```python
from build123d import *

# Parameters (mm, degrees)
SKETCH_1_W          = 120
SKETCH_1_H          = 120
EXTRUDE_1_DEPTH     = 3
SKETCH_3_W          = 123
SKETCH_3_H          = 120
EXTRUDE_2_DEPTH     = 5
SKETCH_5_W          = 15.3
SKETCH_5_H          = 15
CUT_EXTRUDE_2_DEPTH = 3
SKETCH_6_R          = 2.6
CUT_EXTRUDE_3_DEPTH = 87.291656607
SKETCH_7_R          = 5.5
CUT_EXTRUDE_4_DEPTH = 1
SKETCH_8_W          = 92.4
SKETCH_8_H          = 3
CUT_EXTRUDE_5_DEPTH = 3
SKETCH_9_R          = 0.5
CUT_EXTRUDE_6_DEPTH = 3
FILLET_1_R          = 1
FILLET_2_R          = 0.5


with BuildPart() as part:
    # 草图1 → 凸台-拉伸1 (new body)
    with BuildSketch(Plane(origin=(0, 0, 0), x_dir=(1, 0, 0), z_dir=(0, 1, 0))):
        Rectangle(SKETCH_1_W, SKETCH_1_H)
    extrude(amount=EXTRUDE_1_DEPTH)

    # 草图3 → 凸台-拉伸2 (add)
    with BuildSketch(Plane.XZ):
        Rectangle(SKETCH_3_W, SKETCH_3_H)
    extrude(amount=EXTRUDE_2_DEPTH)

    # 草图5 → 切除-拉伸2 (cut)
    with BuildSketch(Plane(origin=(0, 3, 0), x_dir=(1, 0, 0), z_dir=(0, 1, 0))):
        with Locations((-53.85, 52.5)):
            Rectangle(SKETCH_5_W, SKETCH_5_H)
        with Locations((53.85, 52.5)):
            Rectangle(SKETCH_5_W, SKETCH_5_H)
        with Locations((-53.85, -52.5)):
            Rectangle(SKETCH_5_W, SKETCH_5_H)
        with Locations((53.85, -52.5)):
            Rectangle(SKETCH_5_W, SKETCH_5_H)
    extrude(amount=-CUT_EXTRUDE_2_DEPTH, mode=Mode.SUBTRACT)

    # 草图6 → 切除-拉伸3 (cut, through all)
    with BuildSketch(Plane(origin=(0, 3, 0), x_dir=(1, 0, 0), z_dir=(0, 1, 0))):
        with Locations(Location((-53.85, 52.5, 0), (0, 0, 270))):
            Circle(SKETCH_6_R)
        with Locations(Location((53.85, 52.5, 0), (0, 0, 270))):
            Circle(SKETCH_6_R)
        with Locations(Location((-53.85, -52.5, 0), (0, 0, 270))):
            Circle(SKETCH_6_R)
        with Locations(Location((53.85, -52.5, 0), (0, 0, 270))):
            Circle(SKETCH_6_R)
    extrude(amount=-CUT_EXTRUDE_3_DEPTH, mode=Mode.SUBTRACT)

    # 草图7 → 切除-拉伸4 (cut)
    with BuildSketch(Plane.XZ.offset(5)):
        with Locations(Location((-53.85, 52.5, 0), (0, 0, 270))):
            Circle(SKETCH_7_R)
        with Locations(Location((-53.85, -52.5, 0), (0, 0, 270))):
            Circle(SKETCH_7_R)
        with Locations(Location((53.85, 52.5, 0), (0, 0, 270))):
            Circle(SKETCH_7_R)
        with Locations(Location((53.85, -52.5, 0), (0, 0, 270))):
            Circle(SKETCH_7_R)
    extrude(amount=-CUT_EXTRUDE_4_DEPTH, mode=Mode.SUBTRACT)

    # 草图8 → 切除-拉伸5 (cut)
    with BuildSketch(Plane(origin=(0, 3, 0), x_dir=(1, 0, 0), z_dir=(0, 1, 0))):
        with Locations((0, 58.5)):
            Rectangle(SKETCH_8_W, SKETCH_8_H)
        with Locations((0, -58.5)):
            Rectangle(SKETCH_8_W, SKETCH_8_H)
    extrude(amount=-CUT_EXTRUDE_5_DEPTH, mode=Mode.SUBTRACT)

    # 草图9 → 切除-拉伸6 (cut)
    with BuildSketch(Plane(origin=(0, 3, 0), x_dir=(1, 0, 0), z_dir=(0, 1, 0))):
        with Locations((-46.7, 45)):
            Circle(SKETCH_9_R)
        with Locations((46.7, 45)):
            Circle(SKETCH_9_R)
        with Locations((-46.7, -45)):
            Circle(SKETCH_9_R)
        with Locations((46.7, -45)):
            Circle(SKETCH_9_R)
    extrude(amount=-CUT_EXTRUDE_6_DEPTH, mode=Mode.SUBTRACT)

    # 圆角1
    fillet_1_edges = [part.edges().sort_by_distance(p)[0] for p in [
        (47.2, 1.5, -45),
        (-47.2, 1.5, 45),
        (47.2, 1.5, 45),
        (-47.2, 1.5, -45),
    ]]
    fillet(fillet_1_edges, radius=FILLET_1_R)

    # 圆角2
    fillet_2_edges = [part.edges().sort_by_distance(p)[0] for p in [
        (46.2, 1.5, -57),
        (-46.2, 1.5, -57),
        (-46.2, 1.5, 57),
        (46.2, 1.5, 57),
        (60, 1.5, -45),
        (-60, 1.5, 45),
        (60, 1.5, 45),
        (-60, 1.5, -45),
    ]]
    fillet(fillet_2_edges, radius=FILLET_2_R)


solid = part.part
```
For this review, take the finished solid that the model builds, in its own axes (mm). A direction names the side the tool comes from. Coordinates: 2 decimals unless noted, no trailing zeros. Loops run counter-clockwise (first coordinate to the right, second up) from the corner with the lowest first, then second, coordinate; pieces in that order, holes last. Notation, with made-up numbers: (54.25, 74.5) -> (104.25, 74.5) arc R8 ccw to (104.25, 85.5) -> close; hole circle Ø2 at (8, -37.75). An arc over 180 degrees is marked (long way). Return JSON: item names as keys, results as strings. Group by question number.
(1) Consider section C-C, the plane x = 13.5. Give the boundary of the cut face in (y, z), plus the area to 3 significant figures.
(2) Mouldability with a two-part tool opening along Z and no side actions: class faces 5 (the flat face through (-61.5, -2, -1)), 6 (the flat face through (-54, 2, 45)), 7 (the flat face through (51, -4, -54)) as pulls with the +Z half, pulls with the -Z half, needs draft (parallel to the pull), parting line crosses it, or undercut.
(3) Tool access review of faces 1 (the flat face through (51, -4, 51)), 2 (the flat face through (46.2, 2, 51)), 3 (the flat face through (-1, 2, 57)), 4 (the flat face through (-60, 1, 1)): name each direction out of +Z, -Z, +X, -X, +Y, -Y from which nothing blocks a thin tool from reaching the whole face with its end or side.
(4) Consider section B-B, the plane z = -52. Give the boundary of the cut face in (x, y), plus the area to 3 significant figures.
(5) Consider section A-A, the plane x = 53.85. Give the boundary of the cut face in (y, z).
(6) To check wall thickness, follow L1, parallel to X at y = -2, z = -52.5; L2, parallel to X at y = -4.65, z = 52.5; L3, parallel to Z at x = -54.5, y = -3.25. State the ranges of each line that lie inside material, in increasing order.
(7) For pin 1 Ø0.9 at (y, z) = (2, -16) entering from +X; pin 2 Ø9 at (x, z) = (53.85, -52.5) entering from -Y; pin 3 Ø2.5 at (y, z) = (2, -51.5) entering from -X, all flat-tipped, find the tip position at first contact; note any pin that passes through.
Results below:
{
 "1": {"outline": "(-5, -60) -> (0, -60) -> (0, -57) -> (3, -57) -> (3, 57) -> (0, 57) -> (0, 60) -> (-5, 60) -> close", "area": "942 mm2"},
 "2": {"face 5": "needs draft", "face 6": "pulls with the +Z half", "face 7": "undercut"},
 "3": {"face 1": "-Y", "face 2": "+Z, +X, +Y", "face 3": "+Z, +X, -X, +Y", "face 4": "+Z, -Z, -X, +Y"},
 "4": {"outline": "(-61.5, -5) -> (-59.33, -5) -> (-59.33, -4) -> (-56.4, -4) -> (-56.4, 0) -> (-61.5, 0) -> close; (-51.3, -4) -> (-48.37, -4) -> (-48.37, -5) -> (48.37, -5) -> (48.37, -4) -> (51.3, -4) -> (51.3, 0) -> (46.2, 0) -> (46.2, 3) -> (-46.2, 3) -> (-46.2, 0) -> (-51.3, 0) -> close; (56.4, -4) -> (59.33, -4) -> (59.33, -5) -> (61.5, -5) -> (61.5, 0) -> (56.4, 0) -> close", "area": "829 mm2"},
 "5": {"outline": "(-5, -60) -> (0, -60) -> (0, -55.1) -> (-4, -55.1) -> (-4, -58) -> (-5, -58) -> close; (-5, -47) -> (-4, -47) -> (-4, -49.9) -> (0, -49.9) -> (0, -45) -> (3, -45) -> (3, 45) -> (0, 45) -> (0, 49.9) -> (-4, 49.9) -> (-4, 47) -> (-5, 47) -> close; (-5, 58) -> (-4, 58) -> (-4, 55.1) -> (0, 55.1) -> (0, 60) -> (-5, 60) -> close"},
 "6": {"L1": "x = -61.5 to -56.45, -51.25 to 51.25, 56.45 to 61.5", "L2": "x = -61.5 to -59.35, -48.35 to 48.35, 59.35 to 61.5", "L3": "z = -60 to -55.02, -49.98 to 49.98, 55.02 to 60"},
 "7": {"pin 1": "stops at x = 60", "pin 2": "stops at y = -4", "pin 3": "stops at x = -46.2"}
}
